Build history of the part. All positions in model axes, mm. Face numbers are marked on the shaded views. A direction names the side the tool comes from. Give positions to 0.01 mm unless a question says otherwise; leave off trailing zeros. Order: outer loops, then holes, each group sorted by start corner. A loop starts at its lowest first (then second) coordinate and runs counter-clockwise, first axis right, second up. Notation, with made-up numbers: (3, 11) -> (51, 11) arc R36 ccw to (51, 48) -> close; hole circle Ø8 at (85.5, -13.5). An arc over 180 degrees is marked (long way). One line per item, written item: value. Start each with the question number.
(1) Saw through at C-C on x = -18.5. Give the cut face in (y, z), plus the area to 3 significant figures.
(2) Which spindle directions (+Z, -Z, +X, -X, +Y, -Y) get a long thin tool onto all of the face, cutting with end or side? Do the marked faces 4 and 5. Say none if no direction does.
(3) Saw through at B-B on y = 12.5. Give the cut face in (x, z).
(4) Saw through at A-A on z = -6. Give the cut face in (x, y).
(5) Two-plate mould, pull along X, no slides. Class the marked faces 1, 2 and 3: +X half, -X half, draft (parallel to the pull), parting line (faces both ways), or undercut.
(6) Pin check, flat tips, straight feed: pin 1 (9 mm diameter, centred on y = 18.5, z = 10, fed in from +X); pin 2 (4 mm diameter, centred on x = 58, z = -12, fed in from +Y); pin 3 (1.5 mm diameter, centred on y = 30, z = -12, fed in from -X). Stop position of each tip, or through.
(7) Saw through at D-D on x = 6.5. Give the cut face in (y, z).
(8) Probe line 1 (X direction, y = 30.5, z = -16); line 2 (Y direction, x = -57, z = -5); line 3 (Z direction, x = 3, y = 17.5). List the from-to ranges inside material, lowest first.
```python
from build123d import *

# Parameters (mm, degrees)
F0_W     = 127
F0_H     = 50.8
F1_DEPTH = 25.4
F2_W     = 63.5
F2_H     = 50.8
F3_DEPTH = 22.86
F4_W     = 5.08
F4_H     = 5.080003
F4_H_2   = 5.08
F5_DEPTH = 25.4
F6_SIZE  = 1.27
F7_W     = 63.5
F7_H     = 11.43
F8_DEPTH = 62.484


with BuildPart() as f1:
    # F0 (on Top) → F1 (new body)
    with BuildSketch(Plane.XY):
        with Locations((-0.232585, 9.525337)):
            Rectangle(F0_W, F0_H)
    extrude(amount=F1_DEPTH)

    # F2 (on face) → F3 (cut)
    with BuildSketch(Plane.XY.offset(25.4)):
        with Locations((31.517415, 9.525337)):
            Rectangle(F2_W, F2_H)
    extrude(amount=-F3_DEPTH, mode=Mode.SUBTRACT)

    # F4 (on face) → F5 (join)
    with BuildSketch(Plane(origin=(0, 0, 0), x_dir=(1, 0, 0), z_dir=(0, 0, -1))):
        with Locations((-57.216454, 8.838313)):
            Rectangle(F4_W, F4_H)
        with Locations((-57.216454, -30.235119)):
            Rectangle(F4_W, F4_H_2)
        with Locations((56.765015, 8.838313)):
            Rectangle(F4_W, F4_H)
        with Locations((56.765015, -30.235119)):
            Rectangle(F4_W, F4_H_2)
    extrude(amount=F5_DEPTH)

    # F6
    f6_edges = [f1.edges().sort_by_distance(p)[0] for p in [
        (-54.676454, 30.235119, -25.4),
        (-57.216454, 27.695119, -25.4),
        (-59.756454, 30.235119, -25.4),
        (-57.216454, 32.775119, -25.4),
        (59.305015, 30.235119, -25.4),
        (56.765015, 32.775119, -25.4),
        (54.225015, 30.235119, -25.4),
        (56.765015, 27.695119, -25.4),
        (59.305015, -8.838314, -25.4),
        (56.765015, -6.298312, -25.4),
        (54.225015, -8.838314, -25.4),
        (56.765015, -11.378315, -25.4),
        (-54.676454, -8.838314, -25.4),
        (-57.216454, -6.298312, -25.4),
        (-59.756454, -8.838314, -25.4),
        (-57.216454, -11.378315, -25.4),
    ]]
    chamfer(f6_edges, length=F6_SIZE)

    # F7 (on face) → F8 (cut)
    with BuildSketch(Plane.XZ.offset(15.874663)):
        with Locations((-31.982585, 19.685)):
            Rectangle(F7_W, F7_H)
    extrude(amount=-F8_DEPTH, mode=Mode.SUBTRACT)


solid = f1.part
```
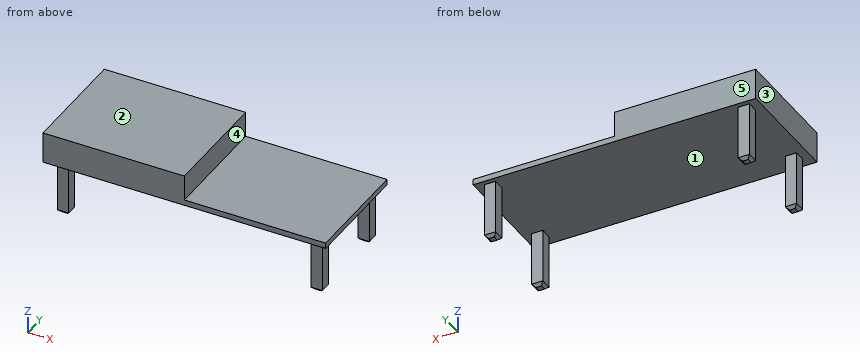
Results below:
1. outline: (-15.87, 0) -> (34.93, 0) -> (34.93, 13.97) -> (-15.87, 13.97) -> close
1. area: 710 mm²
2. face 4: +Z, +X, +Y, -Y
2. face 5: +Z, -Z, +X, -X, +Y
3. outline: (-63.73, 0) -> (63.27, 0) -> (63.27, 2.54) -> (-0.23, 2.54) -> (-0.23, 13.97) -> (-63.73, 13.97) -> close
4. outline: (-59.76, -11.38) -> (-54.68, -11.38) -> (-54.68, -6.3) -> (-59.76, -6.3) -> close; (-59.76, 27.7) -> (-54.68, 27.7) -> (-54.68, 32.78) -> (-59.76, 32.78) -> close; (54.23, -11.38) -> (59.31, -11.38) -> (59.31, -6.3) -> (54.23, -6.3) -> close; (54.23, 27.7) -> (59.31, 27.7) -> (59.31, 32.78) -> (54.23, 32.78) -> close
5. face 1: undercut
5. face 2: draft
5. face 3: -X half
6. pin 1: stops at x = -0.23
6. pin 2: stops at y = 32.78
6. pin 3: stops at x = -59.76
7. outline: (-15.87, 0) -> (34.93, 0) -> (34.93, 2.54) -> (-15.87, 2.54) -> close
8. line 1: x = -59.76 to -54.68, 54.23 to 59.31
8. line 2: y = -11.38 to -6.3, 27.7 to 32.78
8. line 3: z = 0 to 2.54
